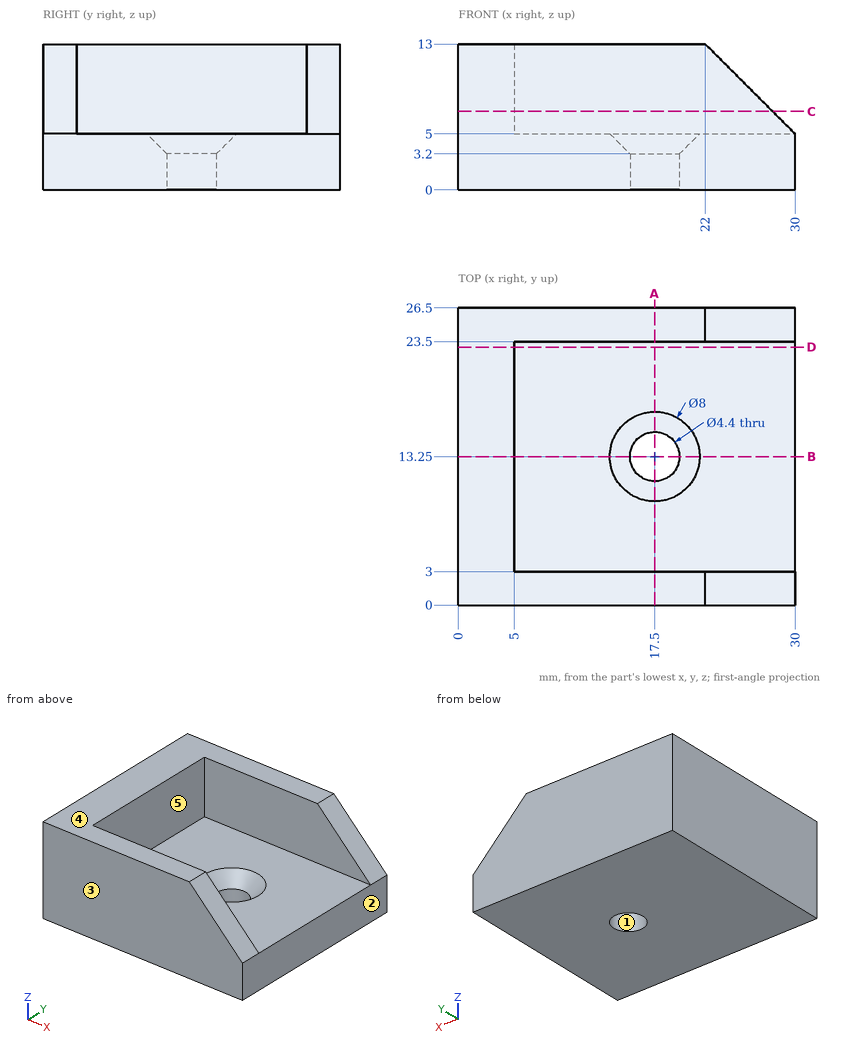
Could you check a few things on this drawing? It's one solid part, dimensions in mm from its lowest x, y, z. A direction names the side the tool comes from. Coordinates: 2 decimals unless noted, no trailing zeros. Order: outer loops, then holes, each group sorted by start corner. A loop starts at its lowest first (then second) coordinate and runs counter-clockwise, first axis right, second up.
1) Will these pins go through, and if not, where does the flat tip stop? pin 1 (4 mm diameter, centred on x = 20, z = 3, fed in from -Y); pin 2 (4 mm diameter, centred on x = 23, y = 14, fed in from +Z); pin 3 (4 mm diameter, centred on y = 16, z = 8.5, fed in from +X).
2) Imagine slicing it at C-C on z = 7. List the corners of the cut face in (x, y) for me, and give its area (4 significant figures).
3) I need wall thicknesses on line 1 (Y direction, x = 12.5, z = 7.25); line 2 (Y direction, x = 17.5, z = 0.8); line 3 (X direction, y = 13.25, z = 1.5). Which ranges of each line are inside material? Lowest first, please.
4) Imagine slicing it at D-D on y = 23. List the corners of the cut face in (x, z) for me.
5) Imagine slicing it at B-B on y = 13.25. List the corners of the cut face in (x, z) for me, and give its area (3 significant figures).
6) Imagine slicing it at A-A on x = 17.5. List the corners of the cut face in (y, z) for me.
7) Which directions (+Z, -Z, +X, -X, +Y, -Y) give clear straight access to the entire face, cutting with the end or side of a thin tool? Please do the marked faces 4 and 5.
8) We'd pull the mould along Y, two halves only. Please class the marked faces 1, 2 and 3: +Y half, -Y half, draft (parallel to the pull), parting line (faces both ways), or undercut.
Response values:
1. pin 1: stops at y = 0
1. pin 2: stops at z = 5
1. pin 3: stops at x = 5
2. outline: (0, 0) - (28, 0) - (28, 3) - (5, 3) - (5, 23.5) - (28, 23.5) - (28, 26.5) - (0, 26.5) - close
2. area: 270.5 mm2
3. line 1: y = 0 to 3, 23.5 to 26.5
3. line 2: y = 0 to 11.05, 15.45 to 26.5
3. line 3: x = 0 to 15.3, 19.7 to 30
4. outline: (0, 0) - (30, 0) - (30, 5) - (5, 5) - (5, 13) - (0, 13) - close
5. outline: (0, 0) - (15.3, 0) - (15.3, 3.2) - (13.5, 5) - (5, 5) - (5, 13) - (0, 13) - close; (19.7, 0) - (30, 0) - (30, 5) - (21.5, 5) - (19.7, 3.2) - close
5. area: 165 mm2
6. outline: (0, 0) - (11.05, 0) - (11.05, 3.2) - (9.25, 5) - (3, 5) - (3, 13) - (0, 13) - close; (15.45, 0) - (26.5, 0) - (26.5, 13) - (23.5, 13) - (23.5, 5) - (17.25, 5) - (15.45, 3.2) - close
7. face 4: +Z, +X, -X, +Y, -Y
7. face 5: +Z, +X
8. face 1: undercut
8. face 2: draft
8. face 3: -Y half
